Autodesk Inventor part; units mm, degrees
ref_plane "YZ Plane" through (0, 0, 0) normal (1, 0, 0) x (0, 1, 0)
ref_plane "XZ Plane" through (0, 0, 0) normal (0, 1, 0) x (-1, 0, 0)
ref_plane "XY Plane" through (0, 0, 0) normal (0, 0, 1) x (1, 0, 0)
sketch "Sketch1" plane through (0, 0, 0) normal (0, 0, 1) x (1, 0, 0)
  circle A0 centre (0, 0) radius 106.3625
  circle A1 centre (0, 0) radius 134.9375
  dimension "d0" = 212.725
  dimension "d1" = 269.875
extrude "Extrusion1" add sketch "Sketch1" along normal blind 1.5875
sketch "Sketch2" plane through (0, 0, 1.5875) normal (0, 0, 1) x (1, 0, 0)
  point P0 (0, 0)
  point P1 (0, 127)
  point P2 (-63.5, 109.9852)
  point P3 (-109.9852, 63.5)
  point P4 (-127, 0)
  point P5 (-109.9852, -63.5)
  point P6 (-63.5, -109.9852)
  point P7 (0, -127)
  point P8 (63.5, -109.9852)
  point P9 (109.9852, -63.5)
  point P10 (127, 0)
  point P11 (109.9852, 63.5)
  point P12 (63.5, 109.9852)
  dimension "d4" = 127
  dimension "d7" = 360
hole "Hole1" at (-63.5, 109.9852, 1.5875) at (-109.9852, 63.5, 1.5875) at (-109.9852, -63.5, 1.5875) at (-63.5, -109.9852, 1.5875) at (63.5, 109.9852, 1.5875) at (109.9852, 63.5, 1.5875) at (109.9852, -63.5, 1.5875) at (63.5, -109.9852, 1.5875) direction (0, 0, -1) diameter 4.9784 end through all
properties part number "3DPRINT,TURRET,SPACER" material "Nylon 6/6"
Can you work these out from the model? Positions are in its coordinate system, mm. Round coordinates to 2 decimals unless told otherwise and drop trailing zeros. Order: outer loops, then holes, each group sorted by start corner. A loop starts at its lowest first (then second) coordinate and runs counter-clockwise, first axis right, second up. Notation, with made-up numbers: M 43,41 L 70,41 A24 cw 70,72 Z; hole C 37.25,-33.5 d3. An arc over 180 degrees is marked long. Use a Markdown table: item, result.
1) Imagine slicing it at B-B (x = -53.5). List the corners of the cut face in (y, z) for me.
Geometry says:
| item | result |
|---|---|
| outline | M -123.88,0 L -91.93,0 L -91.93,1.59 L -123.88,1.59 Z; M 91.93,0 L 123.88,0 L 123.88,1.59 L 91.93,1.59 Z |
2) If I drill on line 1 along X through (y, z) = (1.5, 1.05); line 2 along Y through (x, z) = (0, 1.15); line 3 along Y through (x, z) = (-63.5, 0.75), over which ranges is the centre line in solid material (lowest first)?
Geometry says:
| item | result |
|---|---|
| line 1 | x = -134.93 to -106.35, 106.35 to 134.93 |
| line 2 | y = -134.94 to -106.36, 106.36 to 134.94 |
| line 3 | y = -119.06 to -112.47, -107.5 to -85.33, 85.33 to 107.5, 112.47 to 119.06 |
3) Imagine slicing it at D-D (y = 116). List the corners of the cut face in (x, z) for me.
Geometry says:
| item | result |
|---|---|
| outline | M -68.94,0 L 68.94,0 L 68.94,1.59 L -68.94,1.59 Z |
4) If we mould it in two halves opening along X, with no side actions, what happens to faces 1 (the face through (98.25, 40.74, 0.78)), 2 (the face through (-29.25, 131.73, 0.78)), 3 (the face through (99, 41, 1.588))? For each: +X half, -X half, draft (parallel to the pull), parting line (faces both ways), or undercut.
Geometry says:
| item | result |
|---|---|
| face 1 | undercut |
| face 2 | parting line |
| face 3 | draft |
5) Imagine slicing it at C-C (z = 0.85). Give the number of separate pieces and of enclosed holes in the cut face, then the cut area to 3 significant figures.
Geometry says:
| item | result |
|---|---|
| separate pieces | 1 |
| enclosed holes | 9 |
| area | 21,500 mm² |
6) I'm going to push a flat-ended pin straight in: P1, Ø3, axis at x = -63.5, y = 109.99, coming from the +Z side. Where does the tip first touch, or does it pass through?
Geometry says:
| item | result |
|---|---|
| P1 | passes through |
7) Imagine slicing it at A-A (y = 0). List the corners of the cut face in (x, z) for me, then the cut area to 3 significant figures.
Geometry says:
| item | result |
|---|---|
| outline | M -134.94,0 L -106.36,0 L -106.36,1.59 L -134.94,1.59 Z; M 106.36,0 L 134.94,0 L 134.94,1.59 L 106.36,1.59 Z |
| area | 90.7 mm² |
